from build123d import *

# Parameters (mm, degrees)
EXTRUS_O1_DEPTH                      = 15.24
EXTRUS_O2_DEPTH                      = 3.81
ESBO_O4_R                            = 6.35
EXTRUS_O3_DEPTH                      = 38.1
ESBO_O5_R                            = 17.78
EXTRUS_O4_DEPTH                      = 25.4
ESBO_O6_R                            = 1.778
EXTRUS_O5_DEPTH                      = 25.4
EXTRUS_O6_DEPTH                      = 7.62
ESBO_O8_W                            = 3.175
ESBO_O8_H                            = 3.175
EXTRUS_O8_DEPTH                      = 35.56
FILETE5_R                            = 1.651
FILETE6_R                            = 1.651
CHANFRO1_SIZE                        = 1.27
F_10_32_TAPPED_HOLE3_D               = 4.0386
F_10_32_TAPPED_HOLE3_DEPTH           = 11.938
F_10_32_TAPPED_HOLE3_TIP             = 1.213317848
F_10_32_TAPPED_HOLE3_ON_FACE_2_D     = 4.0386
F_10_32_TAPPED_HOLE3_ON_FACE_2_DEPTH = 11.938
F_10_32_TAPPED_HOLE3_ON_FACE_2_TIP   = 1.213317848
ESBO_O17_R                           = 5.000000033
CORTE_EXTRUS_O1_DEPTH                = 2.54
F_10_32_TAPPED_HOLE1_D               = 4.0386
F_10_32_TAPPED_HOLE1_DEPTH           = 10.0000054
F_10_32_TAPPED_HOLE1_TIP             = 1.213317848
BOSS_EXTRUDE1_DEPTH                  = 0.5
F_10_32_TAPPED_HOLE2_D               = 4.0386
F_10_32_TAPPED_HOLE2_DEPTH           = 11.938
F_10_32_TAPPED_HOLE2_TIP             = 1.213317848
F_6_32_TAPPED_HOLE1_D                = 2.7051
F_6_32_TAPPED_HOLE1_DEPTH            = 9.398
F_6_32_TAPPED_HOLE1_TIP              = 0.81269403
ESBO_O18_W                           = 1
ESBO_O18_H                           = 22.86
ESBO_O18_W_2                         = 22.86
ESBO_O18_H_2                         = 1
CORTE_EXTRUS_O2_DEPTH                = 3.8


with BuildPart() as part:
    # Esboço2 → Extrusão1 (new body)
    with BuildSketch(Plane(origin=(0, 0, 0), x_dir=(0, 0, -1), z_dir=(1, 0, 0))):
        with BuildLine():
            Line((2.54, 0), (35.56, 0))
            ThreePointArc((35.56, 0), (37.356051224, 0.743948776), (38.1, 2.54))
            Line((38.1, 2.54), (38.1, 35.56))
            ThreePointArc((38.1, 35.56), (37.356051224, 37.356051224), (35.56, 38.1))
            Line((35.56, 38.1), (2.54, 38.1))
            ThreePointArc((2.54, 38.1), (0.743948776, 37.356051224), (0, 35.56))
            Line((0, 35.56), (0, 2.54))
            ThreePointArc((0, 2.54), (0.743948776, 0.743948776), (2.54, 0))
        make_face()
    extrude(amount=-EXTRUS_O1_DEPTH)

    # Esboço3 → Extrusão2 (cut)
    with BuildSketch(Plane(origin=(0, 0, 0), x_dir=(0, 0, -1), z_dir=(1, 0, 0))):
        with BuildLine():
            Line((0, 35.56), (0, 30.48))
            Line((0, 30.48), (5.08, 30.48))
            ThreePointArc((5.08, 30.48), (6.876051224, 31.223948776), (7.62, 33.02))
            Line((7.62, 33.02), (7.62, 38.1))
            Line((7.62, 38.1), (2.54, 38.1))
            ThreePointArc((2.54, 38.1), (0.743948776, 37.356051224), (0, 35.56))
        make_face()
        with BuildLine():
            ThreePointArc((0, 2.54), (0.743948776, 0.743948776), (2.54, 0))
            Line((2.54, 0), (7.62, 0))
            Line((7.62, 0), (7.62, 5.08))
            ThreePointArc((7.62, 5.08), (6.876051224, 6.876051224), (5.08, 7.62))
            Line((5.08, 7.62), (0, 7.62))
            Line((0, 7.62), (0, 2.54))
        make_face()
        with BuildLine():
            Line((30.48, 5.08), (30.48, 0))
            Line((30.48, 0), (35.56, 0))
            ThreePointArc((35.56, 0), (37.356051224, 0.743948776), (38.1, 2.54))
            Line((38.1, 2.54), (38.1, 7.62))
            Line((38.1, 7.62), (33.02, 7.62))
            ThreePointArc((33.02, 7.62), (31.223948776, 6.876051224), (30.48, 5.08))
        make_face()
        with BuildLine():
            Line((33.02, 30.48), (38.1, 30.48))
            Line((38.1, 30.48), (38.1, 35.56))
            ThreePointArc((38.1, 35.56), (37.356051224, 37.356051224), (35.56, 38.1))
            Line((35.56, 38.1), (30.48, 38.1))
            Line((30.48, 38.1), (30.48, 33.02))
            ThreePointArc((30.48, 33.02), (31.223948776, 31.223948776), (33.02, 30.48))
        make_face()
    extrude(amount=-EXTRUS_O2_DEPTH, mode=Mode.SUBTRACT)

    # Esboço4 → Extrusão3 (add)
    with BuildSketch(Plane(origin=(0, 0, 0), x_dir=(0, 0, -1), z_dir=(1, 0, 0))):
        with Locations(Location((19.05, 19.05, 0), (0, 0, 180))):
            Circle(ESBO_O4_R)
    extrude(amount=EXTRUS_O3_DEPTH)

    # Esboço5 → Extrusão4 (add)
    with BuildSketch(Plane.ZY.offset(15.24)):
        with Locations(Location((-19.05, 19.05, 0), (0, 0, 180))):
            Circle(ESBO_O5_R)
    extrude(amount=EXTRUS_O4_DEPTH)

    # Esboço6 → Extrusão5 (add)
    with BuildSketch(Plane.ZY.offset(15.24)):
        with Locations(Location((-3.81, 3.81, 0), (0, 0, 180))):
            Circle(ESBO_O6_R)
        with Locations(Location((-34.29, 3.81, 0), (0, 0, 180))):
            Circle(ESBO_O6_R)
        with Locations(Location((-3.81, 34.29, 0), (0, 0, 180))):
            Circle(ESBO_O6_R)
        with Locations(Location((-34.29, 34.29, 0), (0, 0, 180))):
            Circle(ESBO_O6_R)
    extrude(amount=EXTRUS_O5_DEPTH)

    # Esboço7 → Extrusão6 (add)
    with BuildSketch(Plane.ZY.offset(40.64)):
        with BuildLine():
            Line((-2.54, 0), (-35.56, 0))
            ThreePointArc((-35.56, 0), (-37.356051224, 0.743948776), (-38.1, 2.54))
            Line((-38.1, 2.54), (-38.1, 35.56))
            ThreePointArc((-38.1, 35.56), (-37.356051224, 37.356051224), (-35.56, 38.1))
            Line((-35.56, 38.1), (-2.54, 38.1))
            ThreePointArc((-2.54, 38.1), (-0.743948776, 37.356051224), (0, 35.56))
            Line((0, 35.56), (0, 2.54))
            ThreePointArc((0, 2.54), (-0.743948776, 0.743948776), (-2.54, 0))
        make_face()
    extrude(amount=EXTRUS_O6_DEPTH)

    # Esboço8 → Extrusão8 (cut)
    with BuildSketch(Plane(origin=(38.1, 0, 0), x_dir=(0, 0, -1), z_dir=(1, 0, 0))):
        with Locations((12.7, 19.05)):
            Rectangle(ESBO_O8_W, ESBO_O8_H)
    extrude(amount=-EXTRUS_O8_DEPTH, mode=Mode.SUBTRACT)

    # Filete5
    # the kernel refuses this fillet: 1.651 mm, written as the material it adds along each edge
    with BuildSketch(Plane(origin=(2.54, 20.6375, -8.774138938), x_dir=(0, -1, 0), z_dir=(0, 0, -1))) as filete5_piece_1_section:
        with BuildLine():
            CenterArc((FILETE5_R, -FILETE5_R), FILETE5_R, 90, 90)
            Line((0, -FILETE5_R), (0, 0))
            Line((0, 0), (FILETE5_R, 0))
        make_face()
    filete5_piece_1 = extrude(amount=9.640861062, mode=Mode.PRIVATE)
    filete5_piece_1 = filete5_piece_1 & Plane(origin=(2.54, 19.05, -19.05), x_dir=(0, 0, 1), z_dir=(-1, 0, 0)) * Cylinder(6.35, 26, mode=Mode.PRIVATE)
    add(filete5_piece_1)

    # Filete6
    # the kernel refuses this fillet: 1.651 mm, written as the material it adds along each edge
    with BuildSketch(Plane(origin=(2.54, 17.4625, -18.402770343), x_dir=(0, 1, 0), z_dir=(0, 0, 1))) as filete6_piece_1_section:
        with BuildLine():
            CenterArc((1.651, -1.646108137), FILETE6_R, 94.411725786, 85.588274214)
            Line((0, -1.646108137), (-0.03302, -1.646108137))
            Line((-0.03302, -1.646108137), (-0.03302, 0))
            Line((-0.03302, 0), (0, 0.03302))
            ThreePointArc((0, 0.03302), (0.762, 0.03302), (1.52146, 0.032922163))
            Line((1.52146, 0.032922163), (1.524, 0))
        make_face()
    filete6_piece_1 = extrude(amount=9.616401749, mode=Mode.PRIVATE)
    filete6_piece_1 = filete6_piece_1 & Plane(origin=(2.54, 19.05, -19.05), x_dir=(0, 0, 1), z_dir=(-1, 0, 0)) * Cylinder(6.35, 26, mode=Mode.PRIVATE)
    add(filete6_piece_1)

    # Chanfro1
    # the kernel refuses this chamfer: 1.27 mm, written as the material it takes off along each edge
    with BuildSketch(Plane(origin=(38.1, 19.05, -19.05), x_dir=(0, -0.003141587485879291, 0.9999950652018581), z_dir=(0, 0.9999950652018581, 0.003141587485879291))) as chanfro1_piece_1:
        Polygon((6.35, -CHANFRO1_SIZE), (6.35 - CHANFRO1_SIZE, 0), (6.35, 0), align=None)
    revolve(axis=Axis((38.1, 19.05, -19.05), (1, 0, 0)), revolution_arc=359.64, mode=Mode.SUBTRACT)

    # #10-32 Tapped Hole3
    with Locations(Plane(origin=(-7.12, 38.1, -9.54999995), x_dir=(0, 0, 1), z_dir=(0, 1, 0))):
        with Locations((0, 0), (-19.00000005, 0), (-5e-08, -36.83), (-19.0000001, -36.829999984)):
            Hole(F_10_32_TAPPED_HOLE3_D / 2, depth=F_10_32_TAPPED_HOLE3_DEPTH)
            with Locations((0, 0, -(F_10_32_TAPPED_HOLE3_DEPTH + F_10_32_TAPPED_HOLE3_TIP / 2))):  # 118° drill point
                Cone(0, F_10_32_TAPPED_HOLE3_D / 2, F_10_32_TAPPED_HOLE3_TIP, mode=Mode.SUBTRACT)

    # #10-32 Tapped Hole3 on face 2
    with Locations(Plane(origin=(-6.765900445, 0, 15.465533415), x_dir=(0, 0, 1), z_dir=(0, 1, 0))):
        with Locations((0, 0), (-1.090277919, -0.890410597)):
            Hole(F_10_32_TAPPED_HOLE3_ON_FACE_2_D / 2, depth=F_10_32_TAPPED_HOLE3_ON_FACE_2_DEPTH)
            with Locations((0, 0, -(F_10_32_TAPPED_HOLE3_ON_FACE_2_DEPTH + F_10_32_TAPPED_HOLE3_ON_FACE_2_TIP / 2))):  # 118° drill point
                Cone(0, F_10_32_TAPPED_HOLE3_ON_FACE_2_D / 2, F_10_32_TAPPED_HOLE3_ON_FACE_2_TIP, mode=Mode.SUBTRACT)

    # Esboço17 → Corte-extrusão1 (cut)
    with BuildSketch(Plane.ZY.offset(48.26)):
        with Locations((-19.05, 19.05)):
            Circle(ESBO_O17_R)
    extrude(amount=-CORTE_EXTRUS_O1_DEPTH, mode=Mode.SUBTRACT)

    # #10-32 Tapped Hole1
    with Locations(Plane(origin=(38.1, 0, 0), x_dir=(0, 0, -1), z_dir=(1, 0, 0))):
        with Locations((19.05, 19.05)):
            Hole(F_10_32_TAPPED_HOLE1_D / 2, depth=F_10_32_TAPPED_HOLE1_DEPTH)
            with Locations((0, 0, -(F_10_32_TAPPED_HOLE1_DEPTH + F_10_32_TAPPED_HOLE1_TIP / 2))):  # 118° drill point
                Cone(0, F_10_32_TAPPED_HOLE1_D / 2, F_10_32_TAPPED_HOLE1_TIP, mode=Mode.SUBTRACT)

    # Sketch4 → Boss-Extrude1 (add)
    with BuildSketch(Plane(origin=(0, 0, 0), x_dir=(0, 0, -1), z_dir=(1, 0, 0))):
        Polygon((30.48, 0), (7.62, 0), (7.62, 7.62), (0, 7.62), (0, 30.48), (7.62, 30.48), (7.62, 38.1), (30.48, 38.1), (30.48, 30.48), (38.1, 30.48), (38.1, 7.62), (30.48, 7.62), align=None)
    extrude(amount=BOSS_EXTRUDE1_DEPTH)

    # #10-32 Tapped Hole2
    with Locations(Plane.XZ):
        with Locations((-7.12, -9.55), (-7.12, -28.55), (-43.949999984, -9.55), (-43.949999984, -28.55)):
            Hole(F_10_32_TAPPED_HOLE2_D / 2, depth=F_10_32_TAPPED_HOLE2_DEPTH)
            with Locations((0, 0, -(F_10_32_TAPPED_HOLE2_DEPTH + F_10_32_TAPPED_HOLE2_TIP / 2))):  # 118° drill point
                Cone(0, F_10_32_TAPPED_HOLE2_D / 2, F_10_32_TAPPED_HOLE2_TIP, mode=Mode.SUBTRACT)

    # #6-32 Tapped Hole1
    with Locations(Plane(origin=(-3.81, 0, 0), x_dir=(0, 0, -1), z_dir=(1, 0, 0))):
        with Locations((3.975, 34.125), (34.125, 34.125), (3.975, 3.975), (34.125, 3.975)):
            Hole(F_6_32_TAPPED_HOLE1_D / 2, depth=F_6_32_TAPPED_HOLE1_DEPTH)
            with Locations((0, 0, -(F_6_32_TAPPED_HOLE1_DEPTH + F_6_32_TAPPED_HOLE1_TIP / 2))):  # 118° drill point
                Cone(0, F_6_32_TAPPED_HOLE1_D / 2, F_6_32_TAPPED_HOLE1_TIP, mode=Mode.SUBTRACT)

    # Esboço18 → Corte-extrusão2 (cut)
    with BuildSketch(Plane(origin=(0.5, 0, 0), x_dir=(0, 0, -1), z_dir=(1, 0, 0))):
        with Locations((0.5, 19.05)):
            Rectangle(ESBO_O18_W, ESBO_O18_H)
        with Locations((19.05, 37.6)):
            Rectangle(ESBO_O18_W_2, ESBO_O18_H_2)
        with Locations((37.6, 19.05)):
            Rectangle(ESBO_O18_W, ESBO_O18_H)
        with Locations((19.05, 0.5)):
            Rectangle(ESBO_O18_W_2, ESBO_O18_H_2)
    extrude(amount=-CORTE_EXTRUS_O2_DEPTH, mode=Mode.SUBTRACT)


solid = part.part
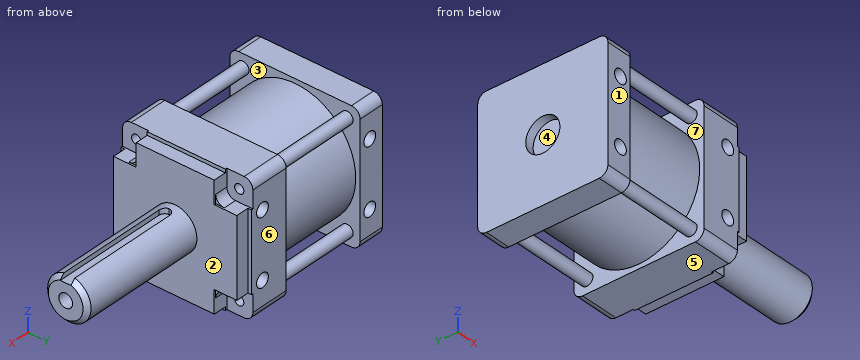
The listing builds one solid part. Answer for the finished solid, in the listing's coordinates (mm). Face numbers are marked on the shaded views. A direction names the side the tool comes from. Give positions to 0.01 mm unless a question says otherwise; leave off trailing zeros. Write each loop counter-clockwise with the first axis right and the second up, starting at its lowest first coordinate (ties: lowest second). Pieces come first, ordered by that corner, then holes. Notation, with made-up numbers: (-20.75, 3) -> (-9.75, 3) arc R15 cw to (-9.75, 21) -> close; hole circle Ø3 at (-19.5, 87). An arc over 180 degrees is marked (long way). Use a Markdown table: item, result.
(1) Find the intervals of material crossed by probe 1 along Z at (x, y) = (-7, 7); probe 2 along Y at (x, z) = (-9, -34); probe 3 along Z at (x, y) = (-11.5, 34.5), in increasing order. Write a range as from..to.
Return value:
| item | result |
|---|---|
| probe 1 | -38.1..-30.57, -26.53..-11.57, -7.53..0 |
| probe 2 | 0..2.63, 5.32..32.78, 35.47..38.1 |
| probe 3 | -38.1..-35.42, -32.83..-5.27, -2.68..0 |
(2) Flat-ended cylindrical pins translate along their axes: P1, Ø9, axis at y = 19.05, z = -19.05, coming from the -X side; P2, Ø2, axis at y = 7, z = -6.5, coming from the +X side; P3, Ø8.5, axis at y = 35, z = -2.5, coming from the +X side. Find the tip coordinate at first contact, or state that the pin passes through.
Return value:
| item | result |
|---|---|
| P1 | x = -45.72 |
| P2 | x = 0.5 |
| P3 | x = -3.81 |
(3) Section C-C, the plane x = 29 is taken. Determine the outline of the cut face in (y, z), then the cut area to 3 significant figures.
Return value:
| item | result |
|---|---|
| outline | (17.46, -14.29) -> (17.46, -12.9) arc R6.35 ccw (long way) to (20.64, -12.9) -> (20.64, -14.29) -> close; hole circle Ø4.04 at (19.05, -19.05) |
| area | 109 mm2 |
(4) Section D-D, the plane y = 6.5 is taken. Determine the outline of the cut face in (x, z).
Return value:
| item | result |
|---|---|
| outline | (-48.26, -38.1) -> (-40.64, -38.1) -> (-40.64, -31.64) -> (-15.24, -31.64) -> (-15.24, -38.1) -> (-3.81, -38.1) -> (-3.81, -30.91) -> (0, -30.91) -> (0, -30.48) -> (0.5, -30.48) -> (0.5, -7.62) -> (0, -7.62) -> (0, -7.19) -> (-3.81, -7.19) -> (-3.81, 0) -> (-15.24, 0) -> (-15.24, -6.46) -> (-40.64, -6.46) -> (-40.64, 0) -> (-48.26, 0) -> close; hole circle Ø4.04 at (-43.95, -28.55); hole circle Ø4.04 at (-43.95, -9.55); hole circle Ø4.04 at (-7.12, -28.55); hole circle Ø4.04 at (-7.12, -9.55) |
(5) Section B-B, the plane y = 11 is taken. Determine the outline of the cut face in (x, z), then the cut area to 3 significant figures.
Return value:
| item | result |
|---|---|
| outline | (-48.26, -38.1) -> (-40.64, -38.1) -> (-40.64, -34.9) -> (-15.24, -34.9) -> (-15.24, -38.1) -> (-3.3, -38.1) -> (-3.3, -37.1) -> (0.5, -37.1) -> (0.5, -1) -> (-3.3, -1) -> (-3.3, 0) -> (-15.24, 0) -> (-15.24, -3.2) -> (-40.64, -3.2) -> (-40.64, 0) -> (-48.26, 0) -> close; hole circle Ø4.04 at (-43.95, -28.55); hole circle Ø4.04 at (-43.95, -9.55); hole circle Ø4.04 at (-7.12, -28.55); hole circle Ø4.04 at (-7.12, -9.55) |
| area | 1,640 mm2 |
(6) For the marked faces 1, 2, 3 and 4, determine the directions among +Z, -Z, +X, -X, +Y, -Y from which every point of the face is accessible in a straight line to the end or side of a thin tool.
Return value:
| item | result |
|---|---|
| face 1 | +Z, -Z, +X, -X, -Y |
| face 2 | +X |
| face 3 | none |
| face 4 | -X |
(7) Section A-A, the plane x = -27.5 is taken. Determine the outline of the cut face in (y, z).
Return value:
| item | result |
|---|---|
| outline | circle Ø35.56 at (19.05, -19.05); circle Ø3.56 at (3.81, -34.29); circle Ø3.56 at (3.81, -3.81); circle Ø3.56 at (34.29, -34.29); circle Ø3.56 at (34.29, -3.81) |
(8) Determine the mould class of the marked faces 5, 6 and 7 for opening direction Z: released by +Z, released by -Z, zero draft, split by the parting line, or undercut.
Return value:
| item | result |
|---|---|
| face 5 | released by -Z |
| face 6 | zero draft |
| face 7 | undercut |
